```python
from build123d import *

# Parameters (mm, degrees)
SKETCH1_W           = 18.9
SKETCH1_H           = 8.5
SKETCH1_W_2         = 4.35
SKETCH1_H_2         = 6.5
BOSS_EXTRUDE1_DEPTH = 5
SKETCH2_W           = 18.9
SKETCH2_H           = 1
BOSS_EXTRUDE2_DEPTH = 10
SKETCH3_R           = 1.4
CUT_EXTRUDE1_DEPTH  = 2


with BuildPart() as part:
    # Sketch1 → Boss-Extrude1 (new body)
    with BuildSketch(Plane(origin=(0, 0, 0), x_dir=(1, 0, 0), z_dir=(0, 1, 0))):
        Rectangle(SKETCH1_W, SKETCH1_H)
        with Locations((-6.275, 0)):
            Rectangle(SKETCH1_W_2, SKETCH1_H_2, mode=Mode.SUBTRACT)
        Rectangle(SKETCH1_W_2, SKETCH1_H_2, mode=Mode.SUBTRACT)
        with Locations((6.275, 0)):
            Rectangle(SKETCH1_W_2, SKETCH1_H_2, mode=Mode.SUBTRACT)
    extrude(amount=BOSS_EXTRUDE1_DEPTH)

    # Sketch2 → Boss-Extrude2 (add)
    with BuildSketch(Plane(origin=(0, 5, 0), x_dir=(1, 0, 0), z_dir=(0, 1, 0))):
        with Locations((0, 3.75)):
            Rectangle(SKETCH2_W, SKETCH2_H)
    extrude(amount=BOSS_EXTRUDE2_DEPTH)

    # Sketch3 → Cut-Extrude1 (cut, through all)
    with BuildSketch(Plane.XY.offset(-3.25)):
        with Locations((7.05, 12.6)):
            Circle(SKETCH3_R)
        with Locations((-7.05, 12.6)):
            Circle(SKETCH3_R)
    extrude(amount=-CUT_EXTRUDE1_DEPTH, mode=Mode.SUBTRACT)


solid = part.part
```
Source: CAD feature listing. Evaluate the final solid. Frame: model axes, mm. A direction names the side the tool comes from. Coordinates: 2 decimals unless noted, no trailing zeros. Loops run counter-clockwise (first coordinate to the right, second up) from the corner with the lowest first, then second, coordinate; pieces in that order, holes last. Notation, with made-up numbers: (17.5, 65) -> (48.5, 65) arc R18 ccw to (48.5, 94) -> close; hole circle Ø11 at (74, 37.5). An arc over 180 degrees is marked (long way). One line per item, written item: value. Start each with the question number.
Q1. Section query A-A, the plane x = -1.5. Return the cut outline in (y, z), and give its area (3 significant figures).
Q2. Contact query for flat-ended pins moving along their axis: P1, Ø1, axis at x = -6, z = 3, coming from the +Y side; P2, Ø5, axis at x = 5.5, y = 13.5, coming from the +Z side. Output: stop coordinate, or through.
Q3. Section query C-C, the plane x = -7.05. Return the cut outline in (y, z), and give its area (3 significant figures).
Q4. Line query: line 1 along Z through (x, y) = (-1.25, 2); line 2 along Y through (x, z) = (-7.05, -3.95); line 3 along Z through (x, y) = (4, 9.75). Output: solid intervals per line, ascending.
Q5. Mould query, pull axis Z, two halves, no side actions, for faces 4 (the face through (0, 15, -4)), 5 (the face through (6, 2, 3.25)), 6 (the face through (0, 2, 4.25)). Classes: pulls with the +Z half, pulls with the -Z half, needs draft (parallel to the pull), parting line crosses it, or undercut.
Q6. Set-up query: faces 1 (the face through (0, 7, -3.25)), 2 (the face through (9.45, 4, -1)), 3 (the face through (-4.1, 2, 0)). Return all of +Z, -Z, +X, -X, +Y, -Y with unobstructed straight access to the full face (end or side cutting, diameter ignored); none if empty.
Q7. Section query D-D, the plane y = 12.6. Return the cut outline in (x, z).
Q8. Section query B-B, the plane z = 2.5. Return the cut outline in (x, y) (3 decimals), and give its area (4 significant figures).
Results:
1. outline: (0, -4.25) -> (15, -4.25) -> (15, -3.25) -> (0, -3.25) -> close; (0, 3.25) -> (5, 3.25) -> (5, 4.25) -> (0, 4.25) -> close
1. area: 20.0 mm^2
2. P1: y = 5
2. P2: z = -3.25
3. outline: (0, -4.25) -> (11.2, -4.25) -> (11.2, -3.25) -> (0, -3.25) -> close; (0, 3.25) -> (5, 3.25) -> (5, 4.25) -> (0, 4.25) -> close; (14, -4.25) -> (15, -4.25) -> (15, -3.25) -> (14, -3.25) -> close
3. area: 17.2 mm^2
4. line 1: -4.25 to -3.25, 3.25 to 4.25
4. line 2: 0 to 11.2, 14 to 15
4. line 3: -4.25 to -3.25
5. face 4: needs draft
5. face 5: undercut
5. face 6: pulls with the +Z half
6. face 1: +Y
6. face 2: +Z, -Z, +X, +Y, -Y
6. face 3: +Y, -Y
7. outline: (-9.45, -4.25) -> (-8.45, -4.25) -> (-8.45, -3.25) -> (-9.45, -3.25) -> close; (-5.65, -4.25) -> (5.65, -4.25) -> (5.65, -3.25) -> (-5.65, -3.25) -> close; (8.45, -4.25) -> (9.45, -4.25) -> (9.45, -3.25) -> (8.45, -3.25) -> close
8. outline: (-9.45, 0) -> (-8.45, 0) -> (-8.45, 5) -> (-9.45, 5) -> close; (-4.1, 0) -> (-2.175, 0) -> (-2.175, 5) -> (-4.1, 5) -> close; (2.175, 0) -> (4.1, 0) -> (4.1, 5) -> (2.175, 5) -> close; (8.45, 0) -> (9.45, 0) -> (9.45, 5) -> (8.45, 5) -> close
8. area: 29.25 mm^2
